Geometry check sheet. Reference: drawing and pictorial views, mm from the part's lowest x, y, z. A direction names the side the tool comes from. Round coordinates to 2 decimals unless told otherwise and drop trailing zeros. Write each loop counter-clockwise with the first axis right and the second up, starting at its lowest first coordinate (ties: lowest second). Pieces come first, ordered by that corner, then holes. Notation, with made-up numbers: M 30,73.25 L 62,73.25 A24 cw 62,89.25 Z; hole C 62.5,57.25 d8. An arc over 180 degrees is marked long. Answer in a Markdown table with one row per item.
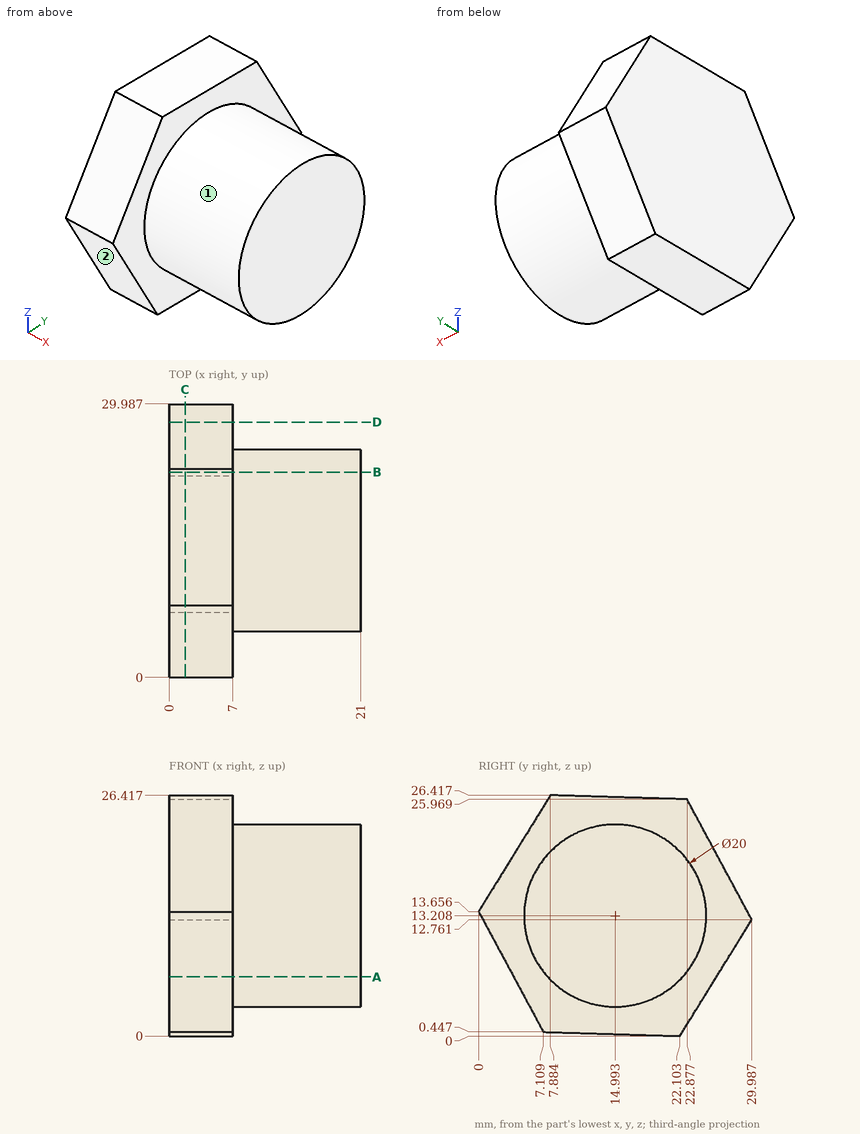
1. Access from +Z, -Z, +X, -X, +Y, -Y to the whole of each face (thin tool, end or side, straight path). Record for the marked faces 1 and 2.
Found:
| item | result |
|---|---|
| face 1 | +X |
| face 2 | -Z, +X, -X, -Y |
2. Scan lines: L1, parallel to Y at x = 16.75, z = 13.25; L2, parallel to X at y = 25, z = 20.5; L3, parallel to Y at x = 6.25, z = 11.75 (1 decimal). Record each from-to range of solid material in increasing order.
Found:
| item | result |
|---|---|
| L1 | y = 4.99 to 24.99 |
| L2 | x = 0 to 7 |
| L3 | y = 1 to 29.4 |
3. Section check D-D, the plane y = 28. Record the cut outline in (x, z) (1 decimal).
Found:
| item | result |
|---|---|
| outline | M 0,9.5 L 7,9.5 L 7,16.5 L 0,16.5 Z |
4. Section check B-B, the plane y = 22.5. Record the cut outline in (x, z) (1 decimal), and give its area (3 significant figures).
Found:
| item | result |
|---|---|
| outline | M 0,0.6 L 7,0.6 L 7,6.6 L 21,6.6 L 21,19.8 L 7,19.8 L 7,26 L 0,26 Z |
| area | 362 mm2 |
5. Section check C-C, the plane x = 1.75. Record the cut outline in (y, z) (1 decimal).
Found:
| item | result |
|---|---|
| outline | M 0,13.7 L 7.1,0.4 L 22.1,0 L 30,12.8 L 22.9,26 L 7.9,26.4 Z |
6. Section check A-A, the plane z = 6.5. Record the cut outline in (x, y).
Found:
| item | result |
|---|---|
| outline | M 0,3.85 L 7,3.85 L 7,7.58 L 21,7.58 L 21,22.41 L 7,22.41 L 7,26.12 L 0,26.12 Z |
7. Go/stop test with flat-tipped pins: pin 1 (4 mm diameter, centred on x = 7.5, z = 23, fed in from +Y); pin 2 (12 mm diameter, centred on x = 3, y = 10, fed in from -Z); pin 3 (10 mm diameter, centred on x = 4, y = 23.5, fed in from +Z). Record where each tip stops, or that it passes through.
Found:
| item | result |
|---|---|
| pin 1 | stops at y = 25.52 |
| pin 2 | stops at z = 0.18 |
| pin 3 | stops at z = 26.1 |
